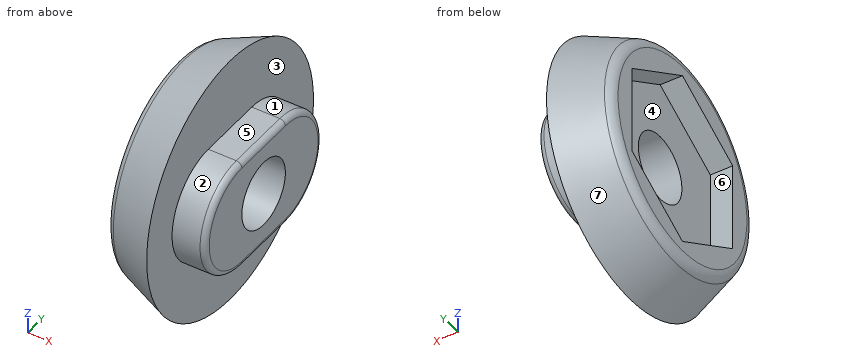
```python
from build123d import *

# Parameters (mm, degrees)
SKETCH_1_W          = 1.7
SKETCH_1_H          = 4.55
FILLET_1_R          = 1
SKETCH_3_R          = 3
EXTRUDE_1_DEPTH     = 3
FILLET_3_R          = 0.5
CUT_EXTRUDE_1_DEPTH = 2


with BuildPart() as part:
    # Эскиз1 → Повернуть1 (revolve)
    with BuildSketch(Plane.XY, mode=Mode.PRIVATE) as revolve_1_sk:
        with Locations((-0.85, 5.275)):
            Rectangle(SKETCH_1_W, SKETCH_1_H)
        Polygon((3, 7.03692641), (3, 3), (0, 3), (0, 7.55), (-1.7, 7.55), (-1.7, 9.55), (3, 11.5), align=None)
    revolve(revolve_1_sk.sketch.rotate(Axis((0, 0, 0), (1, 0, 0)), 90), axis=Axis((0, 0, 0), (1, 0, 0)))

    # Скругление1
    fillet_1_edges = [part.edges().sort_by_distance(p)[0] for p in [
        (-1.7, 0, -9.55),
    ]]
    fillet(fillet_1_edges, radius=FILLET_1_R)

    # Эскиз3 → Бобышка-Вытянуть1 (add)
    with BuildSketch(Plane(origin=(3, 0, 0), x_dir=(0, 0, -1), z_dir=(1, 0, 0))):
        with BuildLine():
            Line((-5, -3), (-5, 3))
            ThreePointArc((-5, 3), (0, 8), (5, 3))
            Line((5, 3), (5, -3))
            ThreePointArc((5, -3), (0, -8), (-5, -3))
        make_face()
        with Locations(Location((0, 0, 0), (0, 0, 180))):
            Circle(SKETCH_3_R, mode=Mode.SUBTRACT)
    extrude(amount=EXTRUDE_1_DEPTH)

    # Скругление3
    fillet_3_edges = [part.edges().sort_by_distance(p)[0] for p in [
        (6, -8, 0),
        (6, 0, -5),
        (6, 8, 0),
        (6, 0, 5),
    ]]
    fillet(fillet_3_edges, radius=FILLET_3_R)

    # Эскиз4 → Вырез-Вытянуть1 (cut)
    with BuildSketch(Plane.ZY.offset(1.7)):
        Polygon((4, 6.92820323), (-4, 6.92820323), (-8, 0), (-4, -6.92820323), (4, -6.92820323), (8, 0), align=None)
    extrude(amount=-CUT_EXTRUDE_1_DEPTH, mode=Mode.SUBTRACT)


solid = part.part
```
Verification items for the finished model (mm, model axes). Face numbers are marked on the shaded views. A direction names the side the tool comes from. Coordinates: 2 decimals unless noted, no trailing zeros. Order: outer loops, then holes, each group sorted by start corner. A loop starts at its lowest first (then second) coordinate and runs counter-clockwise, first axis right, second up. Notation, with made-up numbers: (35, 24.25) - (87, 24.25) arc R25 cw to (87, 59.25) - close; hole circle Ø7 at (23.5, 82). An arc over 180 degrees is marked (long way). Return JSON: item names as keys, results as strings.
(1) Mould release check, pull along Z, two halves, no side actions. Record for the marked faces 4, 5, 6 and 7: pulls with the +Z half, pulls with the -Z half, needs draft (parallel to the pull), parting line crosses it, or undercut.
Filled sheet:
{"face 4": "undercut", "face 5": "pulls with the +Z half", "face 6": "undercut", "face 7": "parting line crosses it"}
(2) Thickness scan on line 1 along X through (y, z) = (3.5, -7.75); line 2 along Y through (x, z) = (3.4, 0); line 3 along X through (y, z) = (3, 3). Record the ranges inside material, lowest first.
Filled sheet:
{"line 1": "x = -1.7 to 3", "line 2": "y = -8 to -3, 3 to 8", "line 3": "x = 0.3 to 6"}
(3) Section check A-A, the plane z = 0. Record the cut outline in (x, y).
Filled sheet:
{"outline": "(-1.7, -8.88) arc R1 ccw to (-1.08, -9.81) - (3, -11.5) - (3, -8) - (5.5, -8) arc R0.5 ccw to (6, -7.5) - (6, -3) - (0.3, -3) - (0.3, -6.93) - (-1.7, -6.93) - close; (-1.7, 6.93) - (0.3, 6.93) - (0.3, 3) - (6, 3) - (6, 7.5) arc R0.5 ccw to (5.5, 8) - (3, 8) - (3, 11.5) - (-1.08, 9.81) arc R1 ccw to (-1.7, 8.88) - close"}
(4) Go/stop test with flat-tipped pins: pin 1 (0.8 mm diameter, centred on x = 5, y = 0.5, fed in from -Z); pin 2 (8 mm diameter, centred on y = 0, z = 0, fed in from -X); pin 3 (0.6 mm diameter, centred on x = -0.5, z = -0.5, fed in from -Y); pin 4 (1 mm diameter, centred on x = 5, z = 6, fed in from -Y). Record where each tip stops, or that it passes through.
Filled sheet:
{"pin 1": "stops at z = -5", "pin 2": "stops at x = 0.3", "pin 3": "stops at y = -10.16", "pin 4": "passes through"}
(5) Section check B-B, the plane x = 4.75. Record the cut outline in (y, z).
Filled sheet:
{"outline": "(-3, -5) - (3, -5) arc R5 ccw to (3, 5) - (-3, 5) arc R5 ccw to start; hole circle Ø6 at (0, 0)"}
(6) Access from +Z, -Z, +X, -X, +Y, -Y to the whole of each face (thin tool, end or side, straight path). Record for the marked faces 1, 2 and 3.
Filled sheet:
{"face 1": "+X, +Y", "face 2": "+X, -Y", "face 3": "+X"}
